Could you check a few things on this model? Use its own coordinates, in mm. A direction names the side the tool comes from. Coordinates: 2 decimals unless noted, no trailing zeros. Loops run counter-clockwise (first coordinate to the right, second up) from the corner with the lowest first, then second, coordinate; pieces in that order, holes last.
Autodesk Inventor part; units mm, degrees
ref_plane "YZ Plane" through (0, 0, 0) normal (1, 0, 0) x (0, 1, 0)
ref_plane "XZ Plane" through (0, 0, 0) normal (0, 1, 0) x (-1, 0, 0)
ref_plane "XY Plane" through (0, 0, 0) normal (0, 0, 1) x (1, 0, 0)
sketch "Sketch1" plane through (0, 0, 0) normal (0, 1, 0) x (-1, 0, 0)
  line L0 (0, 0) -> (24.6, 0)
  line L1 (50, 0) -> (50, -25)
  line L2 (50, -25) -> (24.6, -25)
  line L3 (0, -25) -> (0, 0)
  line L4 (50, 0) -> (24.6, 0) construction
  line L5 (24.6, 0) -> (24.6, -25)
  line L6 (24.6, -25) -> (50, -25) construction
  line L7 (50, -25) -> (50, 0) construction
  line L8 (24.6, 0) -> (50, 0)
  line L9 (24.6, -25) -> (0, -25)
  point P0 (37.3, -12.5)
  dimension "d0" = 50
  dimension "d1" = 25
  dimension "d2" = 25.4
extrude "Extrusion1" add sketch "Sketch1" along normal blind 3 contours L8 L1 L2 L5
hole "Hole1" at (-37.3, 0, -12.5) direction (0, 1, 0) diameter 4.2 end through all
extrude "Extrusion2" add sketch "Sketch1" along normal blind 3 contours L0 L5 L9 L3
extrude "Extrusion3" add sketch "Sketch1" against normal blind 3 contours L0 L5 L9 L3
sketch "Sketch2" plane through (0, 3, 0) normal (1, 0, 0) x (0, 0, -1)
  line L0 (12.5, -0.947) -> (12.5, -4.9651)
  line L1 (25, -3) -> (0, -3)
  point P0 (6.25, -3)
  point P1 (18.75, -3)
hole "Hole2" at (0, 0, -18.75) at (0, 0, -6.25) direction (-1, 0, 0) diameter 2.5 depth 10 tip angle 118
properties part number "Metal_mount_vertical_v1"
(1) Imagine slicing it at B-B, the plane z = -20.5. Write out the boundary of the cut face in (x, y).
Answers:
outline: (-50, 0) - (-24.6, 0) - (-24.6, -3) - (0, -3) - (0, 3) - (-50, 3) - close
(2) Imagine slicing it at D-D, the plane y = -2.35. Write out the boundary of the cut face in (x, z), and give its area (3 significant figures).
Answers:
outline: (-24.6, -25) - (0, -25) - (0, 0) - (-24.6, 0) - close
area: 615 mm2
(3) Imagine slicing it at C-C, the plane x = -43. Write out the boundary of the cut face in (y, z), and give its area (3 significant figures).
Answers:
outline: (0, -25) - (3, -25) - (3, 0) - (0, 0) - close
area: 75.0 mm2
(4) Which directions (+Z, -Z, +X, -X, +Y, -Y) give clear straight access to the entire face, cutting with the end or side of a thin tool? Please do faces 5 (the face through (-37, 0, -10)), 6 (the face through (-5, 0, -5)), 7 (the face through (-20, 1, -25)).
Answers:
face 5: +Z, -Z, -X, -Y
face 6: +X
face 7: -Z, +X, -X, +Y, -Y
(5) For pin 1 (7.5 mm diameter, centred on x = -39, z = -7.5, fed in from -Y); pin 2 (2 mm diameter, centred on y = 0, z = -18.75, fed in from +X); pin 3 (2.5 mm diameter, centred on y = -2, z = -11, fed in from -X), each with a flat end and sliding along its axis, tell me the tip position at first contact or that it passes through.
Answers:
pin 1: stops at y = 0
pin 2: stops at x = -10.15
pin 3: stops at x = -24.6
(6) Imagine slicing it at A-A, the plane z = -12.5. Write out the boundary of the cut face in (x, y), and give its area (3 significant figures).
Answers:
outline: (-50, 0) - (-39.4, 0) - (-39.4, 3) - (-50, 3) - close; (-35.2, 0) - (-24.6, 0) - (-24.6, -3) - (0, -3) - (0, 3) - (-35.2, 3) - close
area: 211 mm2
(7) We'd pull the mould along X, two halves only. Please class faces 1 (the face through (-39.382, 1.521, -12.227)), 2 (the face through (-50, 1, -12)), 3 (the face through (0, 0, -13)), 4 (the face through (-12, -3, -12)): +X half, -X half, draft (parallel to the pull), parting line (faces both ways), or undercut.
Answers:
face 1: undercut
face 2: -X half
face 3: +X half
face 4: draft
(8) I need wall thicknesses on probe 1 along Z at (x, y) = (-2.5, 0); probe 2 along Z at (x, y) = (-37.3, 2.3); probe 3 along Y at (x, z) = (-7.25, -18.75). Which ranges of each line are inside material? Lowest first, please.
Answers:
probe 1: z = -25 to -20, -17.5 to -7.5, -5 to 0
probe 2: z = -25 to -14.6, -10.4 to 0
probe 3: y = -3 to -1.25, 1.25 to 3
